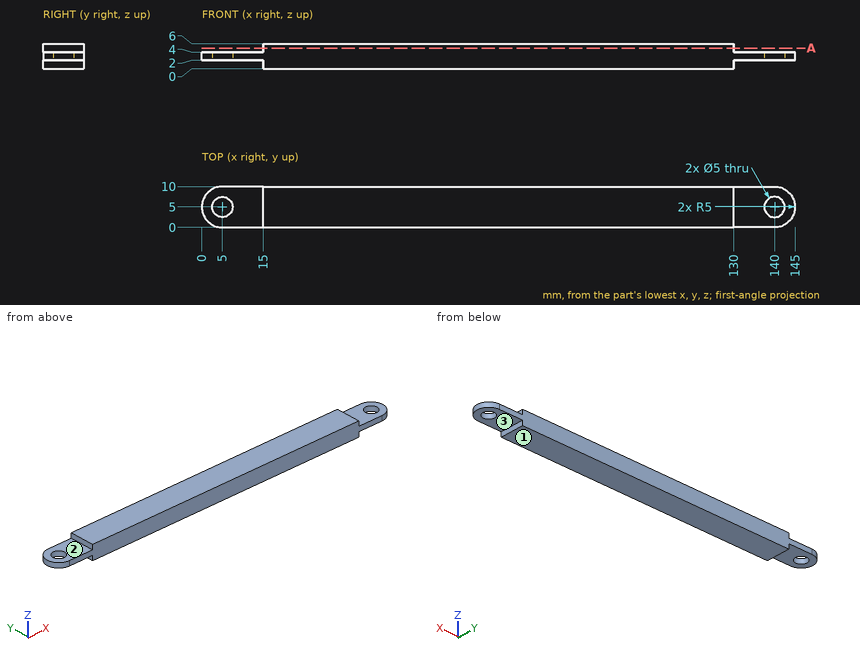
Print and shaded views of the part. All mm, measured from the part's lowest x, y and z. A direction names the side the tool comes from. Coordinates: 2 decimals unless noted, no trailing zeros. Order: outer loops, then holes, each group sorted by start corner. A loop starts at its lowest first (then second) coordinate and runs counter-clockwise, first axis right, second up. Notation, with made-up numbers: (26, 89) - (58, 89) arc R28 cw to (58, 114) - close; hole circle Ø3 at (-1.5, 16). An arc over 180 degrees is marked (long way). Return JSON: item names as keys, results as strings. Group by question number.
Item 1: Drill centre lines: probe 1 along Y at (x, z) = (5, 2.65); probe 2 along X at (y, z) = (6.5, 1.25); probe 3 along X at (y, z) = (2.25, 3.7). Where is each one in solid material? Low to high. Write a range as from..to.
Item 2: Cut at A-A (z = 5). List the corners of the cut face in (x, y), plus the area to 3 significant figures.
Item 3: Which spindle directions (+Z, -Z, +X, -X, +Y, -Y) get a long thin tool onto all of the face, cutting with end or side? Do the marked faces 1, 2 and 3. Say none if no direction does.
Item 4: Pin check, flat tips, straight feed: pin 1 (1 mm diameter, centred on y = 6, z = 5, fed in from +X); pin 2 (2 mm diameter, centred on y = 6.5, z = 1.5, fed in from +X); pin 3 (1 mm diameter, centred on x = 64, z = 2, fed in from -Y); pin 4 (0.6 mm diameter, centred on y = 5.5, z = 4.5, fed in from -X). Stop position of each tip, or through.
Check values:
{
 "1": {"probe 1": "y = 0..2.5, 7.5..10", "probe 2": "x = 15..130", "probe 3": "x = 0.82..144.18"},
 "2": {"outline": "(15, 0) - (130, 0) - (130, 10) - (15, 10) - close", "area": "1,150 mm2"},
 "3": {"face 1": "-Z, +X, -X, +Y, -Y", "face 2": "+Z, -X, +Y, -Y", "face 3": "-Z, +X, +Y, -Y"},
 "4": {"pin 1": "stops at x = 130", "pin 2": "stops at x = 144.96", "pin 3": "stops at y = 0", "pin 4": "stops at x = 15"}
}
